```python
from build123d import *

# Parameters (mm, degrees)
SKETCH1_R           = 2.85
BOSS_EXTRUDE1_DEPTH = 2
SKETCH2_R           = 1.5
BOSS_EXTRUDE2_DEPTH = 8
SKETCH3_W           = 6
SKETCH3_H           = 1
CUT_EXTRUDE1_DEPTH  = 1


with BuildPart() as part:
    # Sketch1 → Boss-Extrude1 (new body)
    with BuildSketch(Plane(origin=(0, 0, 0), x_dir=(1, 0, 0), z_dir=(0, 1, 0))):
        Circle(SKETCH1_R)
    extrude(amount=BOSS_EXTRUDE1_DEPTH)

    # Sketch2 → Boss-Extrude2 (add)
    with BuildSketch(Plane(origin=(0, 0, 0), x_dir=(1, 0, 0), z_dir=(0, 1, 0))):
        Circle(SKETCH2_R)
    extrude(amount=-BOSS_EXTRUDE2_DEPTH)

    # Sketch3 → Cut-Extrude1 (cut)
    with BuildSketch(Plane(origin=(0, 2, 0), x_dir=(1, 0, 0), z_dir=(0, 1, 0))):
        Rectangle(SKETCH3_W, SKETCH3_H)
    extrude(amount=-CUT_EXTRUDE1_DEPTH, mode=Mode.SUBTRACT)


solid = part.part
```
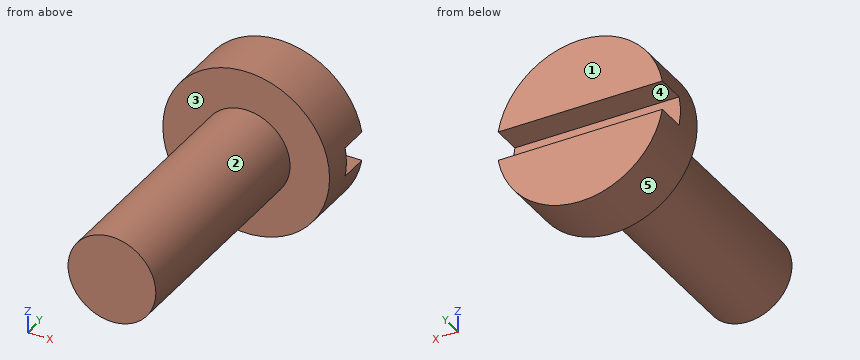
Build history of the part. All positions in model axes, mm. Face numbers are marked on the shaded views. A direction names the side the tool comes from. Give positions to 0.01 mm unless a question says otherwise; leave off trailing zeros. Loops run counter-clockwise (first coordinate to the right, second up) from the corner with the lowest first, then second, coordinate; pieces in that order, holes last. Notation, with made-up numbers: (6.5, 55) -> (38.5, 55) arc R10 ccw to (38.5, 69) -> close; hole circle Ø1 at (38.5, 75.5). An arc over 180 degrees is marked (long way). One line per question, with ' | ' between items. Start each with the question number.
1) Cut at A-A (x = 0). Give the cut face in (y, z), plus the area to 3 significant figures.
2) Two-plate mould, pull along Z, no slides. Class the marked faces 3, 4 and 5: released by +Z, released by -Z, zero draft, split by the parting line, or undercut.
3) Probe L1, parallel to Y at x = -0.2, z = 2.5; L2, parallel to X at y = -4.5, z = -0.1; L3, parallel to Y at x = 1.35, z = -0.25. List the from-to ranges inside material, lowest first.
4) Cut at D-D (z = 0.7). Give the cut face in (x, y).
5) Cut at C-C (y = -3.5). Give the cut face in (x, z).
6) 3-axis set-ups, long thin cutter, end or side, ignore diameter. For the marked faces 1 and 2: which of +Z, -Z, +X, -X, +Y, -Y reach the whole face in a straight line?
7) Cut at B-B (z = 0). Give the cut face in (x, y).
8) Pin check, flat tips, straight feed: pin 1 (3 mm diameter, centred on x = -1.5, y = -4.5, fed in from -Z); pin 2 (0.5 mm diameter, centred on x = 1.5, y = 1.5, fed in from -Z); pin 3 (1.5 mm diameter, centred on y = -4, z = 1, fed in from -X). Stop position of each tip, or through.
Return value:
1) outline: (-8, -1.5) -> (0, -1.5) -> (0, -2.85) -> (2, -2.85) -> (2, -0.5) -> (1, -0.5) -> (1, 0.5) -> (2, 0.5) -> (2, 2.85) -> (0, 2.85) -> (0, 1.5) -> (-8, 1.5) -> close | area: 34.4 mm^2
2) face 3: zero draft | face 4: undercut | face 5: split by the parting line
3) L1: 0 to 2 | L2: -1.5 to 1.5 | L3: -8 to 1
4) outline: (-2.76, 0) -> (-1.33, 0) -> (-1.33, -8) -> (1.33, -8) -> (1.33, 0) -> (2.76, 0) -> (2.76, 2) -> (-2.76, 2) -> close
5) outline: circle Ø3 at (0, 0)
6) face 1: +Z, -Z, +X, -X, +Y | face 2: -Y
7) outline: (-2.85, 0) -> (-1.5, 0) -> (-1.5, -8) -> (1.5, -8) -> (1.5, 0) -> (2.85, 0) -> (2.85, 1) -> (-2.85, 1) -> close
8) pin 1: z = -1.5 | pin 2: z = -2.56 | pin 3: x = -1.48
